Read the model definition and answer for the solid it produces. Units are mm, in the model's axes. Face numbers are marked on the shaded views. A direction names the side the tool comes from. Give positions to 0.01 mm unless a question says otherwise; leave off trailing zeros. Write each loop counter-clockwise with the first axis right and the second up, starting at its lowest first coordinate (ties: lowest second). Pieces come first, ordered by that corner, then holes. Notation, with made-up numbers: M -12.5,67 L 27.5,67 A20 ccw 27.5,91 Z; hole C 15,-2.75 d5. An arc over 180 degrees is marked long. Answer as CSV lines item,"result". Start each with the question number.
```python
from build123d import *

# Parameters (mm, degrees)
SKETCH1_R                = 12.5
SKETCH1_R_2              = 4
BOSS_EXTRUDE1_DEPTH      = 6.5
CUT_EXTRUDE1_DEPTH       = 5.5
CUT_EXTRUDE2_START       = -5.5
CUT_EXTRUDE2_DEPTH       = 5.5
SKETCH5_R                = 12.5
SKETCH5_R_2              = 10.5
CUT_EXTRUDE3_DEPTH       = 2
CUT_EXTRUDE4_START       = -2
SKETCH6_R                = 12.5
SKETCH6_R_2              = 10.5
CUT_EXTRUDE4_DEPTH       = 2
CUT_EXTRUDE5_START       = -13
SKETCH7_R                = 10.5
CUT_EXTRUDE5_DEPTH       = 13
SKETCH8_R                = 2.5
CUT_EXTRUDE6_DEPTH       = 13
CUT_EXTRUDE7_DEPTH       = 1
CUT_EXTRUDE8_START       = -1
CUT_EXTRUDE8_DEPTH       = 1
CUT_EXTRUDE9_START       = -1
CUT_EXTRUDE9_DEPTH       = 1
CUT_EXTRUDE10_DEPTH      = 45.138985036
CUT_EXTRUDE10_DEPTH_BACK = 1
CUT_EXTRUDE11_START      = -1
CUT_EXTRUDE11_DEPTH      = 1
CUT_EXTRUDE12_DEPTH      = 45.138985036
CUT_EXTRUDE12_DEPTH_BACK = 1


# Read off the part's stored shape, not the designer's step: Cut-Extrude9, Cut-Extrude11
with BuildPart() as part:
    # Sketch1 → Boss-Extrude1 (new, symmetric)
    # profile 1 of 10: a face of its own
    with BuildSketch(Plane.XY):
        Circle(SKETCH1_R)
        with Locations(Location((0, 0, 0), (0, 0, 180))):
            Circle(SKETCH1_R_2, mode=Mode.SUBTRACT)
    # profile 2 of 10: a face of its own
    with BuildSketch(Plane.XY):
        with BuildLine():
            ThreePointArc((-13.5, 0), (-13.247641299, -2.598076211), (-12.5, -5.099019514))
            Line((-12.5, -5.099019514), (-12.5, 0))
            ThreePointArc((-12.5, 0), (0, 12.5), (12.5, 0))
            Line((12.5, 0), (12.5, -5.099019514))
            ThreePointArc((12.5, -5.099019514), (13.247641299, -2.598076211), (13.5, 0))
            ThreePointArc((13.5, 0), (0, 13.5), (-13.5, 0))
        make_face()
    # profile 3 of 10: a face of its own
    with BuildSketch(Plane.XY):
        with BuildLine():
            Line((-12.5, 0), (-12.5, -5.099019514))
            ThreePointArc((-12.5, -5.099019514), (0, -13.5), (12.5, -5.099019514))
            Line((12.5, -5.099019514), (12.5, 0))
            ThreePointArc((12.5, 0), (0, -12.5), (-12.5, 0))
        make_face()
    # profile 4 of 10: a face of its own
    with BuildSketch(Plane.XY):
        with BuildLine():
            ThreePointArc((-13.5, 0), (-13.247641299, -2.598076211), (-12.5, -5.099019514))
            Line((-12.5, -5.099019514), (-12.5, 0))
            ThreePointArc((-12.5, 0), (0, 12.5), (12.5, 0))
            Line((12.5, 0), (12.5, -5.099019514))
            ThreePointArc((12.5, -5.099019514), (13.247641299, -2.598076211), (13.5, 0))
            ThreePointArc((13.5, 0), (0, 13.5), (-13.5, 0))
        make_face()
    # profile 5 of 10: a face of its own
    with BuildSketch(Plane.XY):
        with BuildLine():
            Line((-12.5, 0), (-12.5, -5.099019514))
            ThreePointArc((-12.5, -5.099019514), (0, -13.5), (12.5, -5.099019514))
            Line((12.5, -5.099019514), (12.5, 0))
            ThreePointArc((12.5, 0), (0, -12.5), (-12.5, 0))
        make_face()
    # profile 6 of 10: a face of its own
    with BuildSketch(Plane.XY):
        with BuildLine():
            Line((-13.5, -10), (-12.5, -10))
            Line((-12.5, -10), (-12.5, -5.099019514))
            ThreePointArc((-12.5, -5.099019514), (-13.247641299, -2.598076211), (-13.5, 0))
            Line((-13.5, 0), (-13.5, -10))
        make_face()
    # profile 7 of 10: a face of its own
    with BuildSketch(Plane.XY):
        Polygon((-12.5, -14.03581164), (-12.5, -10), (-13.5, -10), (-27.5, -10), (-27.5, -15), (-12.5, -15), align=None)
    # profile 8 of 10: a face of its own
    with BuildSketch(Plane.XY):
        with BuildLine():
            Line((-12.5, -5.099019514), (-12.5, -10))
            Line((-12.5, -10), (-12.5, -14.03581164))
            Line((-12.5, -14.03581164), (12.5, -14.03581164))
            Line((12.5, -14.03581164), (12.5, -10))
            Line((12.5, -10), (12.5, -5.099019514))
            ThreePointArc((12.5, -5.099019514), (0, -13.5), (-12.5, -5.099019514))
        make_face()
    # profile 9 of 10: a face of its own
    with BuildSketch(Plane.XY):
        Polygon((12.5, -10), (12.5, -14.03581164), (12.5, -15), (27.5, -15), (27.5, -10), (13.5, -10), align=None)
    # profile 10 of 10: a face of its own
    with BuildSketch(Plane.XY):
        with BuildLine():
            ThreePointArc((13.5, 0), (13.247641299, -2.598076211), (12.5, -5.099019514))
            Line((12.5, -5.099019514), (12.5, -10))
            Line((12.5, -10), (13.5, -10))
            Line((13.5, -10), (13.5, 0))
        make_face()
    extrude(amount=BOSS_EXTRUDE1_DEPTH, both=True)

    # Sketch3 → Cut-Extrude1 (cut)
    with BuildSketch(Plane.XY.offset(6.5)):
        with BuildLine():
            Line((-12.5, 0), (-12.5, -14.03581164))
            Line((-12.5, -14.03581164), (12.5, -14.03581164))
            Line((12.5, -14.03581164), (12.5, 0))
            ThreePointArc((12.5, 0), (0, -12.5), (-12.5, 0))
        make_face()
    extrude(amount=-CUT_EXTRUDE1_DEPTH, mode=Mode.SUBTRACT)

    # Sketch4 → Cut-Extrude2 (cut)
    with BuildSketch(Plane(origin=(0, 0, -6.5), x_dir=(-1, 0, 0), z_dir=(0, 0, -1)).offset(CUT_EXTRUDE2_START)):
        with BuildLine():
            Line((-12.5, 0), (-12.5, -14.03581164))
            Line((-12.5, -14.03581164), (12.5, -14.03581164))
            Line((12.5, -14.03581164), (12.5, 0))
            ThreePointArc((12.5, 0), (0, -12.5), (-12.5, 0))
        make_face()
    extrude(amount=CUT_EXTRUDE2_DEPTH, mode=Mode.SUBTRACT)

    # Sketch5 → Cut-Extrude3 (cut)
    with BuildSketch(Plane.XY.offset(6.5)):
        Circle(SKETCH5_R)
        Circle(SKETCH5_R_2, mode=Mode.SUBTRACT)
    extrude(amount=-CUT_EXTRUDE3_DEPTH, mode=Mode.SUBTRACT)

    # Sketch6 → Cut-Extrude4 (cut)
    with BuildSketch(Plane(origin=(0, 0, -6.5), x_dir=(-1, 0, 0), z_dir=(0, 0, -1)).offset(CUT_EXTRUDE4_START)):
        Circle(SKETCH6_R)
        with Locations(Location((0, 0, 0), (0, 0, 180))):
            Circle(SKETCH6_R_2, mode=Mode.SUBTRACT)
    extrude(amount=CUT_EXTRUDE4_DEPTH, mode=Mode.SUBTRACT)

    # Sketch7 → Cut-Extrude5 (cut)
    with BuildSketch(Plane(origin=(0, 0, -6.5), x_dir=(-1, 0, 0), z_dir=(0, 0, -1)).offset(CUT_EXTRUDE5_START)):
        Circle(SKETCH7_R)
    extrude(amount=CUT_EXTRUDE5_DEPTH, mode=Mode.SUBTRACT)

    # Sketch8 → Cut-Extrude6 (cut)
    with BuildSketch(Plane(origin=(0, -10, 0), x_dir=(1, 0, 0), z_dir=(0, 1, 0))):
        with Locations(Location((20.5, 0, 0), (0, 0, 180))):
            Circle(SKETCH8_R)
        with Locations(Location((-20.5, 0, 0), (0, 0, 180))):
            Circle(SKETCH8_R)
    extrude(amount=-CUT_EXTRUDE6_DEPTH, mode=Mode.SUBTRACT)

    # Sketch10 → Cut-Extrude7 (cut)
    with BuildSketch(Plane.XY.offset(6.5)):
        with BuildLine():
            Line((-13.5, 0), (-12.5, 0))
            ThreePointArc((-12.5, 0), (0, 12.5), (12.5, 0))
            Line((12.5, 0), (13.5, 0))
            ThreePointArc((13.5, 0), (0, 13.5), (-13.5, 0))
        make_face()
    extrude(amount=-CUT_EXTRUDE7_DEPTH, mode=Mode.SUBTRACT)

    # Sketch11 → Cut-Extrude8 (cut)
    with BuildSketch(Plane(origin=(0, 0, -6.5), x_dir=(-1, 0, 0), z_dir=(0, 0, -1)).offset(CUT_EXTRUDE8_START)):
        with BuildLine():
            Line((-13.5, 0), (-12.5, 0))
            ThreePointArc((-12.5, 0), (0, 12.5), (12.5, 0))
            Line((12.5, 0), (13.5, 0))
            ThreePointArc((13.5, 0), (0, 13.5), (-13.5, 0))
        make_face()
    extrude(amount=CUT_EXTRUDE8_DEPTH, mode=Mode.SUBTRACT)

    # Cut-Extrude9 outline → Cut-Extrude9 (cut)
    with BuildSketch(Plane(origin=(13.5, 0, 0), x_dir=(0, 0, -1), z_dir=(1, 0, 0)).offset(CUT_EXTRUDE9_START)):
        Polygon((-6.5, 0), (-6.5, -10), (-5.5, 0), align=None)
    extrude(amount=CUT_EXTRUDE9_DEPTH, mode=Mode.SUBTRACT)

    # Sketch13 → Cut-Extrude10 (cut, two sides: drawn at the far end of the back side and taken through both)
    with BuildSketch(Plane(origin=(13.5, 0, 0), x_dir=(0, 0, -1), z_dir=(1, 0, 0)).offset(-CUT_EXTRUDE10_DEPTH_BACK)):
        Polygon((6.5, 0), (5.5, 0), (6.5, -10), align=None)
    extrude(amount=CUT_EXTRUDE10_DEPTH + CUT_EXTRUDE10_DEPTH_BACK, mode=Mode.SUBTRACT)

    # Cut-Extrude11 outline → Cut-Extrude11 (cut)
    with BuildSketch(Plane.ZY.offset(13.5).offset(CUT_EXTRUDE11_START)):
        Polygon((-6.5, 0), (-6.5, -10), (-5.5, 0), align=None)
    extrude(amount=CUT_EXTRUDE11_DEPTH, mode=Mode.SUBTRACT)

    # Sketch15 → Cut-Extrude12 (cut, two sides: drawn at the far end of the back side and taken through both)
    with BuildSketch(Plane.ZY.offset(13.5).offset(-CUT_EXTRUDE12_DEPTH_BACK)):
        Polygon((6.5, 0), (5.5, 0), (6.5, -10), align=None)
    extrude(amount=CUT_EXTRUDE12_DEPTH + CUT_EXTRUDE12_DEPTH_BACK, mode=Mode.SUBTRACT)


solid = part.part
```
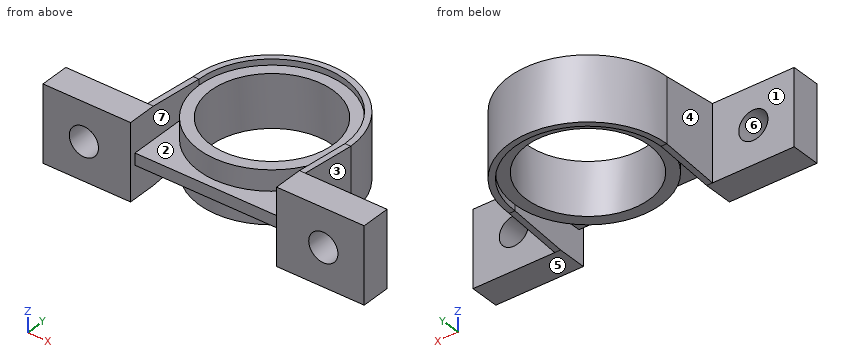
1. Find section A-A on z = 0. Determine the outline of the cut face in (x, y).
2. Find section B-B on x = -20.5. Determine the outline of the cut face in (y, z), then the cut area to 3 significant figures.
3. Find section D-D on x = 0. Determine the outline of the cut face in (y, z).
4. Given pin 1 (3 mm diameter, centred on y = -6.5, z = -2.5, fed in from -X); pin 2 (11 mm diameter, centred on x = 5, y = -6.5, fed in from -Z); pin 3 (6.5 mm diameter, centred on x = -21, z = 2, fed in from +Y); pin 4 (3 mm diameter, centred on x = 20.5, z = 0, fed in from +Y), each flat-ended and moving along its own axis, determine where each tip first touches the part or whether it passes through.
5. Find section C-C on y = 4. Determine the outline of the cut face in (x, z).
6. Determine the mould class of the marked faces 4, 5, 6 and 7 for opening direction X: +X half, -X half, draft (parallel to the pull), parting line (faces both ways), or undercut.
7. For the marked faces 1, 2 and 3, determine the directions among +Z, -Z, +X, -X, +Y, -Y from which every point of the face is accessible in a straight line to the end or side of a thin tool.
8. Find the intervals of material crossed by line 1 (X direction, y = 0.25, z = 3.5); line 2 (Z direction, x = 20.5, y = -12.3); line 3 (Y direction, x = 0, z = -2.25), in increasing order. Write a range as [from, to].
Computed:
1,outline,"M -27.5,-15 L -23,-15 L -23,-10 L -27.5,-10 Z; M -18,-15 L -12.5,-15 L -12.5,-14.04 L 12.5,-14.04 L 12.5,-15 L 18,-15 L 18,-10 L 13.5,-10 L 13.5,0 A13.5 ccw -13.5,0 L -13.5,-10 L -18,-10 Z; M 23,-15 L 27.5,-15 L 27.5,-10 L 23,-10 Z; hole C 0,0 d21"
2,outline,"M -15,-6.5 L -10,-6.5 L -10,-2.5 L -15,-2.5 Z; M -15,2.5 L -10,2.5 L -10,6.5 L -15,6.5 Z"
2,area,"40.0 mm^2"
3,outline,"M -14.04,-1 L -12.5,-1 L -12.5,-4.5 L -10.5,-4.5 L -10.5,4.5 L -12.5,4.5 L -12.5,1 L -14.04,1 Z; M 10.5,-4.5 L 12.5,-4.5 L 12.5,-5.5 L 13.5,-5.5 L 13.5,5.5 L 12.5,5.5 L 12.5,4.5 L 10.5,4.5 Z"
4,pin 1,"stops at x = -13.5"
4,pin 2,"stops at z = -4.5"
4,pin 3,"stops at y = -10"
4,pin 4,"passes through"
5,outline,"M -12.89,-5.5 L -11.84,-5.5 L -11.84,-4.5 L -9.71,-4.5 L -9.71,4.5 L -11.84,4.5 L -11.84,5.5 L -12.89,5.5 Z; M 9.71,-4.5 L 11.84,-4.5 L 11.84,-5.5 L 12.89,-5.5 L 12.89,5.5 L 11.84,5.5 L 11.84,4.5 L 9.71,4.5 Z"
6,face 4,"-X half"
6,face 5,"draft"
6,face 6,"undercut"
6,face 7,"undercut"
7,face 1,"+Z, -Z, -X, +Y"
7,face 2,"+Z, -Y"
7,face 3,"+Z, -Z, +X, +Y"
8,line 1,"x = [-13.5, -10.5], [10.5, 13.5]"
8,line 2,"z = [-6.5, -2.5], [2.5, 6.5]"
8,line 3,"y = [-12.5, -10.5], [10.5, 13.5]"
